```python
from build123d import *

# Parameters (mm, degrees)
F2_R = 2
F3_R = 5


with BuildPart() as f1:
    # F0 (on Front) → F1 (revolve)
    with BuildSketch(Plane.XZ):
        with BuildLine():
            ThreePointArc((-7.0685046336, 10.3095219212), (4.6853520259, 11.5886788028), (12.2474487139, 2.5))
            Line((12.2474487139, 2.5), (74.2474487139, 2.5))
            Line((74.2474487139, 2.5), (80.4566636234, 6.848955093))
            ThreePointArc((80.4566636234, 6.848955093), (71.1861926887, 12.2493617225), (61.3018820008, 8.0772608919))
            add(Edge.make_bspline(
                [(13.7809895682, 12.3177978136), (18.9431640709, 3.8047084098), (45.8510372203, 7.5452258089), (55.5286329868, 6.7225269235), (61.3018820008, 8.0772608919)],
                knots=[0, 0, 0, 0, 0.5718996335, 1, 1, 1, 1], degree=3))
            ThreePointArc((13.7809895682, 12.3177978136), (2.4835532955, 18.3159979112), (-10.003236638, 15.5428141988))
            Line((-10.003236638, 15.5428141988), (-7.0685046336, 10.3095219212))
        make_face()
    revolve(axis=Axis((35, 0, 0), (1, 0, 0)))

    # F2
    f2_edges = [f1.edges().sort_by_distance(p)[0] for p in [
        (80.456664, 0, -6.848955),
        (-7.068505, 0, -10.309522),
        (12.247449, 0, -2.5),
    ]]
    fillet(f2_edges, radius=F2_R)

    # F3
    f3_edges = [f1.edges().sort_by_distance(p)[0] for p in [
        (74.247449, 0, -2.5),
    ]]
    fillet(f3_edges, radius=F3_R)


solid = f1.part
```
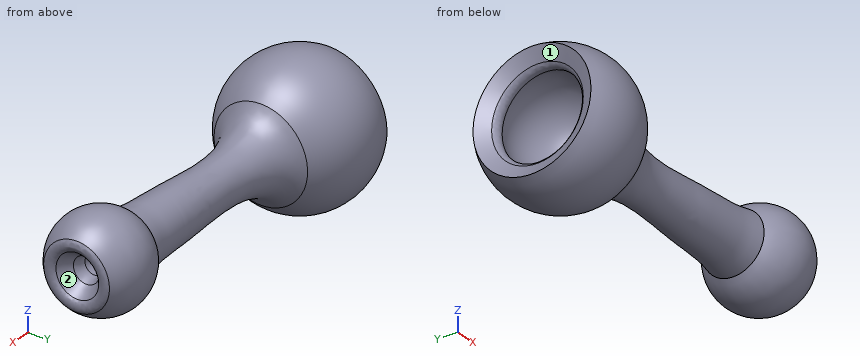
Check sheet for the modelled part. Datum: model origin and axes. Units: mm. Face numbers are marked on the shaded views. Round coordinates to 2 decimals unless told otherwise and drop trailing zeros. Use CSV: the item, a comma, the result in double quotes.
(1) Depth check by flat-ended pin: pin 1 (6.5 mm diameter, centred on y = 0, z = 0, fed in from +X); pin 2 (4 mm diameter, centred on x = 45, z = 0.5, fed in from +Y); pin 3 (12 mm diameter, centred on y = -6, z = -14.5, fed in from +X). Enter the tip coordinate at first touch or a pass-through.
Worked out:
pin 1,"x = 75.3"
pin 2,"y = 6.75"
pin 3,"x = 77.85"
(2) Material ranges on line 1 along Z through (x, y) = (4, -2.5); line 2 along X through (y, z) = (-10.5, -4.5); line 3 along Y through (x, z) = (32.5, 0), recorded low to high. Write a range as from..to.
Worked out:
line 1,"-17.87..-11.58, 11.58..17.87"
line 2,"-7.47..-5.07, 5.07..14.39, 65.98..74.85"
line 3,"-5.88..-2.5, 2.5..5.88"
(3) Draft check along Z on the marked faces 1 and 2. Enter one of: pulls with the +Z half, pulls with the -Z half, needs draft (parallel to the pull), parting line crosses it, or undercut.
Worked out:
face 1,"undercut"
face 2,"undercut"
